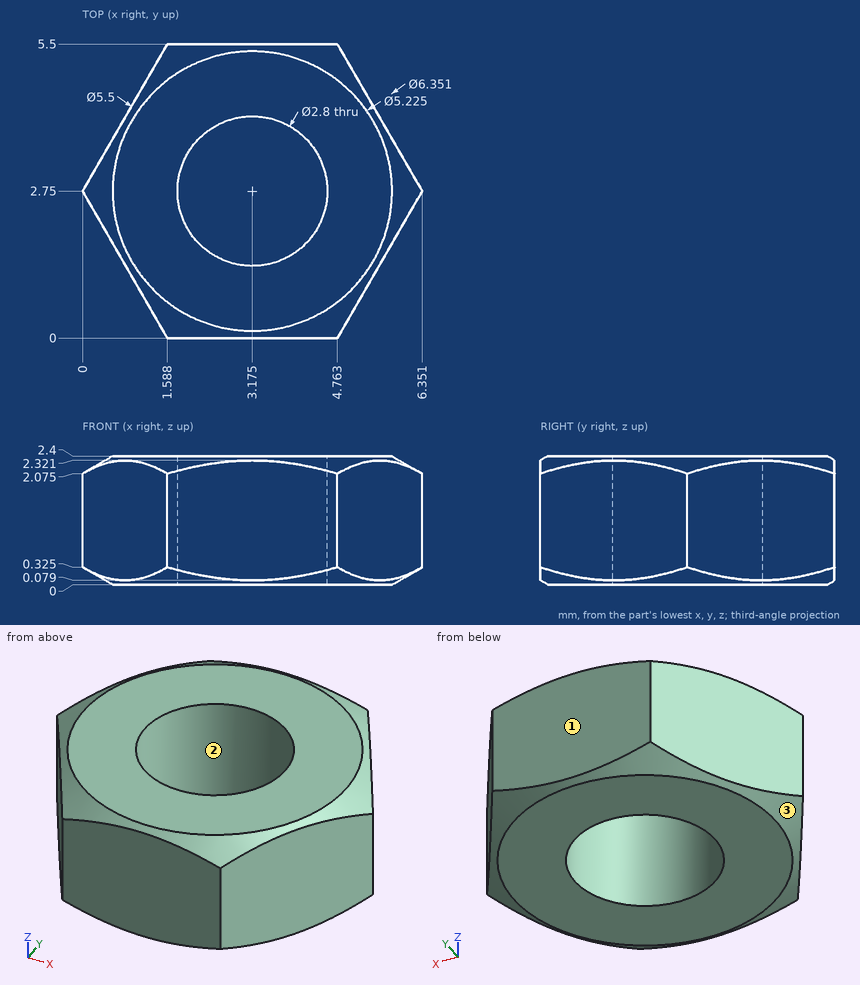
Verification items for this drawing (mm, ordinates from the low corner). Give positions to 0.01 mm unless a question says otherwise; leave off trailing zeros. Answer as a JSON object with one key per item and string values. Group by question number.
Q1. Release check for a two-part mould opening along X. For the marked faces 1, 2 and 3 record: released by +X, released by -X, zero draft, split by the parting line, or undercut.
Q2. Material ranges on line 1 along X through (y, z) = (1.55, 1.65) (1 decimal); line 2 along Y through (x, z) = (2.75, 1.45) (1 decimal); line 3 along Y through (x, z) = (2.5, 2.25) (1 decimal), recorded low to high. Write a range as [from, to].
Q3. Go/stop test with a flat-tipped pin: P1, Ø1, axis at y = 4, z = 0.5, coming from the +X side. Record where the tip stops, or that it passes through.
Evaluation:
{
 "1": {"face 1": "zero draft", "face 2": "undercut", "face 3": "split by the parting line"},
 "2": {"line 1": "x = [0.7, 2.5], [3.9, 5.7]", "line 2": "y = [0, 1.4], [4.1, 5.5]", "line 3": "y = [0, 1.5], [4, 5.5]"},
 "3": {"P1": "stops at x = 5.92"}
}
